from build123d import *

# Parameters (mm, degrees)
BOSS_EXTRUDE2_DEPTH = 3
SKETCH3_R           = 1.5
SKETCH3_W           = 40
SKETCH3_H           = 3
SKETCH3_W_2         = 9
SKETCH3_H_2         = 9
CUT_EXTRUDE1_DEPTH  = 195.996345243
FILLET1_R           = 10
SKETCH4_R           = 1.5
CUT_EXTRUDE2_DEPTH  = 195.996345243
FILLET2_R           = 5


with BuildPart() as part:
    # Sketch2 → Boss-Extrude2 (new body)
    with BuildSketch(Plane.XY):
        Polygon((-80, 167.804878049), (-80, 137.804878049), (-60, 137.804878049), (-60, 93.804878049), (-80, 93.804878049), (-80, 41.804878049), (-60, 41.804878049), (-60, -2.195121951), (-80, -2.195121951), (-80, -12.195121951), (-70, -22.195121951), (70, -22.195121951), (80, -12.195121951), (80, -2.195121951), (60, -2.195121951), (60, 41.804878049), (80, 41.804878049), (80, 93.804878049), (60, 93.804878049), (60, 137.804878049), (80, 137.804878049), (80, 167.804878049), (70, 177.804878049), (-70, 177.804878049), align=None)
    extrude(amount=BOSS_EXTRUDE2_DEPTH)

    # Sketch3 → Cut-Extrude1 (cut, through all)
    with BuildSketch(Plane.XY.offset(3)):
        with Locations((-75, 74.804878049)):
            Circle(SKETCH3_R)
        with Locations((-75, 60.804878049)):
            Circle(SKETCH3_R)
        with Locations((75, 74.804878049)):
            Circle(SKETCH3_R)
        with Locations((75, 60.804878049)):
            Circle(SKETCH3_R)
        with Locations((-34, -7.195121951)):
            Circle(SKETCH3_R)
        with Locations((41, -7.195121951)):
            Circle(SKETCH3_R)
        with Locations((41, 40.804878049)):
            Circle(SKETCH3_R)
        with Locations((-41, 40.804878049)):
            Circle(SKETCH3_R)
        with Locations((-12, 35.804878049)):
            Circle(SKETCH3_R)
        with Locations((-12, 7.804878049)):
            Circle(SKETCH3_R)
        with Locations((-45, 94.804878049)):
            Circle(SKETCH3_R)
        with Locations((-7, 94.804878049)):
            Circle(SKETCH3_R)
        with Locations((-7, 56.804878049)):
            Circle(SKETCH3_R)
        with Locations((-45, 56.804878049)):
            Circle(SKETCH3_R)
        with Locations((-36, 150.804878049)):
            Circle(SKETCH3_R)
        with Locations((36, 150.804878049)):
            Circle(SKETCH3_R)
        with Locations((-7, 172.804878049)):
            Circle(SKETCH3_R)
        with Locations((7, 172.804878049)):
            Circle(SKETCH3_R)
        with Locations((0, -17.695121951)):
            Rectangle(SKETCH3_W, SKETCH3_H)
        with Locations((27.5, 145.304878049)):
            Rectangle(SKETCH3_W_2, SKETCH3_H_2)
    extrude(amount=-CUT_EXTRUDE1_DEPTH, mode=Mode.SUBTRACT)

    # Fillet1
    fillet1_edges = [part.edges().sort_by_distance(p)[0] for p in [
        (-70, 177.804878049, 1.5),
        (70, 177.804878049, 1.5),
        (80, 167.804878049, 1.5),
        (80, -12.195121951, 1.5),
        (70, -22.195121951, 1.5),
        (-70, -22.195121951, 1.5),
        (-80, -12.195121951, 1.5),
        (-80, 167.804878049, 1.5),
    ]]
    fillet(fillet1_edges, radius=FILLET1_R)

    # Sketch4 → Cut-Extrude2 (cut, through all)
    with BuildSketch(Plane.XY.offset(3)):
        with Locations((-70, 85.804878049)):
            Circle(SKETCH4_R)
        with Locations((70, 85.804878049)):
            Circle(SKETCH4_R)
        with Locations((-70, -14.195121951)):
            Circle(SKETCH4_R)
        with Locations((70, -14.195121951)):
            Circle(SKETCH4_R)
    extrude(amount=-CUT_EXTRUDE2_DEPTH, mode=Mode.SUBTRACT)

    # Fillet2
    fillet2_edges = [part.edges().sort_by_distance(p)[0] for p in [
        (80, 137.804878049, 1.5),
        (80, 93.804878049, 1.5),
        (80, 41.804878049, 1.5),
        (80, -2.195121951, 1.5),
        (-80, -2.195121951, 1.5),
        (-80, 41.804878049, 1.5),
        (-80, 93.804878049, 1.5),
        (-80, 137.804878049, 1.5),
    ]]
    fillet(fillet2_edges, radius=FILLET2_R)


solid = part.part
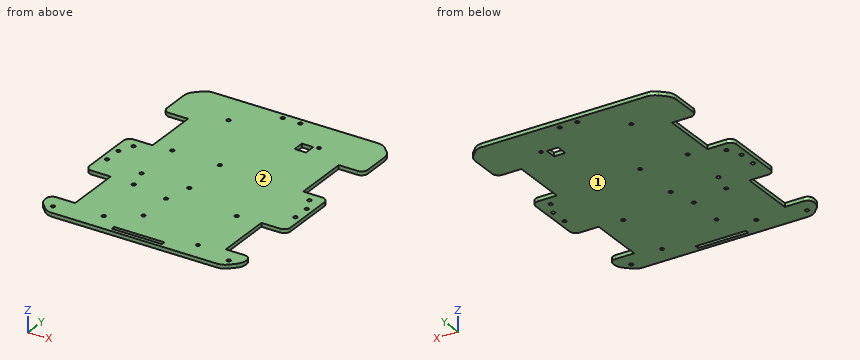
Design review of the part built by this model. Coordinates are the model's own, in mm. Face numbers are marked on the shaded views. Give positions to 0.01 mm unless a question says otherwise; leave off trailing zeros. Write each loop counter-clockwise with the first axis right and the second up, starting at its lowest first coordinate (ties: lowest second). Pieces come first, ordered by that corner, then holes. Notation, with made-up numbers: M 36,56.5 L 68,56.5 A18 ccw 68,71.5 Z; hole C -8.75,19.5 d6. An arc over 180 degrees is marked long. Return JSON: item names as keys, results as strings. Group by question number.
Item 1: The part is to be moulded in two halves that separate along Z. For the marked faces 1 and 2, say which applies: pulls with the +Z half, pulls with the -Z half, needs draft (parallel to the pull), parting line crosses it, or undercut.
Item 2: Clearance check with flat-ended pins moving along their axes: pin 1 Ø1 at (y, z) = (42, 1.5) entering from -X; pin 2 Ø0.9 at (y, z) = (27.5, 2) entering from -X; pin 3 Ø0.9 at (y, z) = (116, 1.5) entering from +X. State where each tip first meets the part, or that it passes through.
Item 3: Take a section at A-A (y = 15). Give the boundary of the cut face in (x, z), plus the area to 3 significant figures.
Item 4: Wall thickness on line 1 along Y through (x, z) = (-7, 2.25); line 2 along X through (y, z) = (86, 1.35); line 3 along Y through (x, z) = (64.5, 2.1): over which ranges is each line inside the solid? List them lowest first.
Item 5: Take a section at B-B (z = 1.65). Count the separate pieces of the cut face and the enclosed holes in it, plus the area to 3 significant figures.
Return value:
{
 "1": {"face 1": "pulls with the -Z half", "face 2": "pulls with the +Z half"},
 "2": {"pin 1": "stops at x = -77.54", "pin 2": "stops at x = -60", "pin 3": "stops at x = 60"},
 "3": {"outline": "M -60,0 L 60,0 L 60,3 L -60,3 Z", "area": "360 mm2"},
 "4": {"line 1": "y = -22.2 to -19.2, -16.2 to 55.3, 58.3 to 93.3, 96.3 to 171.3, 174.3 to 177.8", "line 2": "x = -80 to -71.49, -68.51 to 68.51, 71.49 to 80", "line 3": "y = -22.2 to -2.2, 41.8 to 93.8, 137.8 to 177.8"},
 "5": {"separate pieces": "1", "enclosed holes": "24", "area": "27,900 mm2"}
}
